Build history of the part. All positions in model axes, mm. A direction names the side the tool comes from. Round coordinates to 2 decimals unless told otherwise and drop trailing zeros. Write each loop counter-clockwise with the first axis right and the second up, starting at its lowest first coordinate (ties: lowest second). Pieces come first, ordered by that corner, then holes. Notation, with made-up numbers: (55, 41.25) -> (113, 41.25) arc R13 ccw to (113, 61.25) -> close; hole circle Ø9 at (-8, 68.5). An arc over 180 degrees is marked (long way). One line per question, with ' | ' between items.
from build123d import *

# Parameters (mm, degrees)
SKETCH_1_W               = 84
SKETCH_1_H               = 60
EXTRUDE_1_DEPTH          = 39
SKETCH_3_R               = 36.5
EXTRUDE_2_DEPTH          = 5
SKETCH_4_R               = 1.45
CUT_EXTRUDE_2_DEPTH      = 5
PATTERN_CIRCULAR_1_COUNT = 8
SKETCH_2_W               = 58.75
SKETCH_2_H               = 28.5
CUT_EXTRUDE_1_DEPTH      = 34
SKETCH_6_R               = 10.5
SKETCH_6_R_2             = 2.4
CUT_EXTRUDE_3_DEPTH      = 5
SKETCH_7_R               = 2
CUT_EXTRUDE_4_DEPTH      = 40
SKETCH_8_R               = 3
CUT_EXTRUDE_5_DEPTH      = 34
SKETCH_9_W               = 11
SKETCH_9_H               = 10
CUT_EXTRUDE_6_DEPTH      = 100


with BuildPart() as part:
    # 草图1 → 凸台-拉伸1 (new body)
    with BuildSketch(Plane.XY):
        with Locations((8.550148957, -9.437934459)):
            Rectangle(SKETCH_1_W, SKETCH_1_H)
    extrude(amount=EXTRUDE_1_DEPTH)

    # 草图3 → 凸台-拉伸2 (add)
    with BuildSketch(Plane(origin=(0, 0, 0), x_dir=(-1, 0, 0), z_dir=(0, 0, -1))):
        with Locations((-14.050148957, -9.437934459)):
            Circle(SKETCH_3_R)
    extrude(amount=-EXTRUDE_2_DEPTH)

    # 草图4 → 切除-拉伸2 (cut)
    with BuildSketch(Plane(origin=(0, 0, 0), x_dir=(-1, 0, 0), z_dir=(0, 0, -1))):
        with Locations((-46.550148957, -9.437934459)):
            Circle(SKETCH_4_R)
    cut_extrude_2 = extrude(amount=-CUT_EXTRUDE_2_DEPTH, mode=Mode.SUBTRACT)

    # 阵列(圆周)1: 切除-拉伸2 ×8 about axis
    pattern_circular_1_axis = Axis((14.050148957, -9.437934459, 0), (0, 0, 1))
    for i in range(1, PATTERN_CIRCULAR_1_COUNT):
        add(cut_extrude_2.rotate(pattern_circular_1_axis, i * 360 / PATTERN_CIRCULAR_1_COUNT), mode=Mode.SUBTRACT)

    # 草图2 → 切除-拉伸1 (cut)
    with BuildSketch(Plane(origin=(0, 0, 0), x_dir=(-1, 0, 0), z_dir=(0, 0, -1))):
        with Locations((4.074851043, -9.437934459)):
            Rectangle(SKETCH_2_W, SKETCH_2_H)
    extrude(amount=-CUT_EXTRUDE_1_DEPTH, mode=Mode.SUBTRACT)

    # 草图6 → 切除-拉伸3 (cut)
    with BuildSketch(Plane(origin=(0, 0, 34), x_dir=(-1, 0, 0), z_dir=(0, 0, -1))):
        with Locations((-14.050148957, -9.437934459)):
            Circle(SKETCH_6_R)
        with Locations((-22.050148957, 1.562065541)):
            Circle(SKETCH_6_R_2)
        with Locations((-22.050148957, -20.437934459)):
            Circle(SKETCH_6_R_2)
        with Locations((17.949851043, -20.437934459)):
            Circle(SKETCH_6_R_2)
        with Locations((17.949851043, 1.562065541)):
            Circle(SKETCH_6_R_2)
    extrude(amount=-CUT_EXTRUDE_3_DEPTH, mode=Mode.SUBTRACT)

    # 草图7 → 切除-拉伸4 (cut)
    with BuildSketch(Plane.XY.offset(39)):
        with Locations((-23.449851043, 9.562065541)):
            Circle(SKETCH_7_R)
        with Locations((-23.449851043, -28.437934459)):
            Circle(SKETCH_7_R)
        with Locations((1.550148957, 9.562065541)):
            Circle(SKETCH_7_R)
        with Locations((1.550148957, -28.437934459)):
            Circle(SKETCH_7_R)
    extrude(amount=-CUT_EXTRUDE_4_DEPTH, mode=Mode.SUBTRACT)

    # 草图8 → 切除-拉伸5 (cut)
    with BuildSketch(Plane(origin=(0, 0, 0), x_dir=(-1, 0, 0), z_dir=(0, 0, -1))):
        with Locations((-1.550148957, 9.562065541)):
            Circle(SKETCH_8_R)
        with Locations((23.449851043, 9.562065541)):
            Circle(SKETCH_8_R)
        with Locations((-1.550148957, -28.437934459)):
            Circle(SKETCH_8_R)
        with Locations((23.449851043, -28.437934459)):
            Circle(SKETCH_8_R)
    extrude(amount=-CUT_EXTRUDE_5_DEPTH, mode=Mode.SUBTRACT)

    # 草图9 → 切除-拉伸6 (cut)
    with BuildSketch(Plane(origin=(0, -39.437934459, 0), x_dir=(-1, 0, 0), z_dir=(0, -1, 0))):
        with Locations((0.199851043, -29)):
            Rectangle(SKETCH_9_W, SKETCH_9_H)
    extrude(amount=-CUT_EXTRUDE_6_DEPTH, mode=Mode.SUBTRACT)


solid = part.part
(1) Slice it at A-A (y = 18). Write the cut outline in (x, z).
Calculated:
outline: (-33.45, 0) -> (50.55, 0) -> (50.55, 39) -> (-33.45, 39) -> close; hole (-5.7, 24) -> (5.3, 24) -> (5.3, 34) -> (-5.7, 34) -> close
(2) Mould opens along Y. For faces 1 (the flat face through (0, -32, 24)), 2 (the cylindrical face through (13.74, 27.06, 2.46)), 3 (the flat face through (8, -39.438, 19)), 4 (the flat face through (-10, -9, 34)) say: pulls with the +Y half, pulls with the -Y half, needs draft (parallel to the pull), parting line crosses it, or undercut.
Calculated:
face 1: needs draft | face 2: pulls with the +Y half | face 3: pulls with the -Y half | face 4: undercut
(3) Slice it at B-B (z = 28). Write the cut outline in (x, y).
Calculated:
outline: (-33.45, -39.44) -> (-5.7, -39.44) -> (-5.7, -23.69) -> (-33.45, -23.69) -> close; (-33.45, 4.81) -> (-5.7, 4.81) -> (-5.7, 20.56) -> (-33.45, 20.56) -> close; (5.3, -39.44) -> (50.55, -39.44) -> (50.55, 20.56) -> (5.3, 20.56) -> (5.3, 4.81) -> (25.3, 4.81) -> (25.3, -23.69) -> (5.3, -23.69) -> close; hole circle Ø6 at (-23.45, -28.44); hole circle Ø6 at (-23.45, 9.56)
(4) Wall check: line 1 (Y direction, x = -6.5, z = 28.5); line 2 (X direction, y = -36, z = 28); line 3 (Y direction, x = -26, z = 3). Give the ranges that are in metal, low to high. Write a range as from..to.
Calculated:
line 1: -39.44..-23.69, 4.81..20.56 | line 2: -33.45..-5.7, 5.3..50.55 | line 3: -39.44..-30.02, -26.86..-23.69, 4.81..7.98, 11.14..20.56
(5) Slice it at D-D (y = -15). Write the cut outline in (x, z), then the cut area to 3 significant figures.
Calculated:
outline: (-33.45, 34) -> (5.14, 34) -> (5.14, 39) -> (-33.45, 39) -> close; (22.96, 34) -> (25.3, 34) -> (25.3, 0) -> (50.55, 0) -> (50.55, 39) -> (22.96, 39) -> close | area: 1,190 mm2
(6) 3-axis set-ups, long thin cutter, end or side, ignore diameter. For faces 5 (the cylindrical face through (47.62, -8.46, 2.46)), 6 (the flat face through (5.3, 13, 29)), 7 (the flat face through (14, -40, 5)): which of +Z, -Z, +X, -X, +Y, -Y reach the whole face in a straight line?
Calculated:
face 5: -Z | face 6: +Y, -Y | face 7: +Z, +X, -X, -Y
(7) Slice it at C-C (x = 9.5). Write the cut outline in (y, z), then the cut area to 3 significant figures.
Calculated:
outline: (-45.65, 0) -> (-23.69, 0) -> (-23.69, 34) -> (-18.9, 34) -> (-18.9, 39) -> (-39.44, 39) -> (-39.44, 5) -> (-45.65, 5) -> close; (0.02, 34) -> (4.81, 34) -> (4.81, 0) -> (26.78, 0) -> (26.78, 5) -> (20.56, 5) -> (20.56, 39) -> (0.02, 39) -> close | area: 1,340 mm2
(8) Drop flat-ended pins along their axis: pin 1 (8 mm diameter, centred on x = 23.5, y = -6.5, fed in from +Z); pin 2 (1.5 mm diameter, centred on x = 36.5, y = -32.5, fed in from -Z); pin 3 (2 mm diameter, centred on x = -5, z = 11.5, fed in from +Y); pin 4 (6 mm diameter, centred on x = -17.95, y = -20.44, fed in from -Z). Give the stop position or say it passes through.
Calculated:
pin 1: z = 39 | pin 2: z = 5 | pin 3: y = 20.56 | pin 4: z = 34
